Source: CAD feature listing. Evaluate the final solid. Frame: model axes, mm. Face numbers are marked on the shaded views. A direction names the side the tool comes from. Give positions to 0.01 mm unless a question says otherwise; leave off trailing zeros. Write each loop counter-clockwise with the first axis right and the second up, starting at its lowest first coordinate (ties: lowest second). Pieces come first, ordered by that corner, then holes. Notation, with made-up numbers: M 33.25,21 L 69.25,21 A31 cw 69.25,58 Z; hole C 23,32 d3. An arc over 180 degrees is marked long. Return JSON: item names as keys, results as strings.
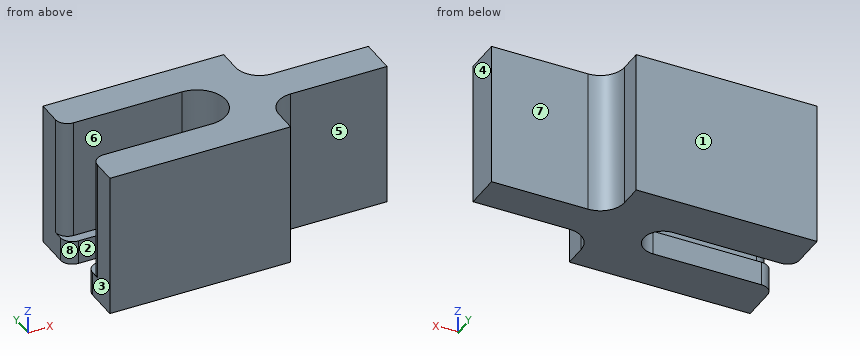
```python
from build123d import *

# Parameters (mm, degrees)
BOSS_EXTRUDE1_DEPTH      = 10
BOSS_EXTRUDE1_DEPTH_BACK = 2
BOSS_EXTRUDE2_START      = -2
BOSS_EXTRUDE2_DEPTH      = 2
FILLET6_R                = 1
FILLET7_R                = 1
BOSS_EXTRUDE3_DEPTH      = 10
BOSS_EXTRUDE3_DEPTH_BACK = 2
SKETCH1_5_W              = 7.906812167
SKETCH1_5_H              = 3
SKETCH1_5_W_2            = 2.093187833
FILLET8_R                = 2


with BuildPart() as part:
    # Sketch1 → Boss-Extrude1 (new, two sides: drawn at the far end of the back side and taken through both)
    with BuildSketch(Plane.XY.offset(-BOSS_EXTRUDE1_DEPTH_BACK)):
        with BuildLine():
            Line((-10, 2.4), (0, 2.4))
            ThreePointArc((0, 2.4), (2.4, 0), (0, -2.4))
            Line((0, -2.4), (-10, -2.4))
            Line((-10, -2.4), (-10, -5.4))
            Line((-10, -5.4), (5, -5.4))
            Line((5, -5.4), (5, -1.5))
            Line((5, -1.5), (5, 1.5))
            Line((5, 1.5), (5, 5.4))
            Line((5, 5.4), (-10, 5.4))
            Line((-10, 5.4), (-10, 2.4))
        make_face()
    extrude(amount=BOSS_EXTRUDE1_DEPTH + BOSS_EXTRUDE1_DEPTH_BACK)

    # Sketch1_4 → Boss-Extrude2 (add)
    with BuildSketch(Plane.XY.offset(BOSS_EXTRUDE2_START)):
        with BuildLine():
            Line((0, 1.6), (-10, 1.6))
            Line((-10, 1.6), (-10, 2.4))
            Line((-10, 2.4), (0, 2.4))
            ThreePointArc((0, 2.4), (2.4, 0), (0, -2.4))
            Line((0, -2.4), (-10, -2.4))
            Line((-10, -2.4), (-10, -1.6))
            Line((-10, -1.6), (0, -1.6))
            ThreePointArc((0, -1.6), (1.6, 0), (0, 1.6))
        make_face()
        with BuildLine():
            Line((-10, 2.4), (0, 2.4))
            ThreePointArc((0, 2.4), (2.4, 0), (0, -2.4))
            Line((0, -2.4), (-10, -2.4))
            Line((-10, -2.4), (-10, -5.4))
            Line((-10, -5.4), (5, -5.4))
            Line((5, -5.4), (5, -1.5))
            Line((5, -1.5), (5, 1.5))
            Line((5, 1.5), (5, 5.4))
            Line((5, 5.4), (-10, 5.4))
            Line((-10, 5.4), (-10, 2.4))
        make_face()
    extrude(amount=BOSS_EXTRUDE2_DEPTH)

    # Fillet6
    fillet6_edges = [part.edges().sort_by_distance(p)[0] for p in [
        (-10, -2.4, 5),
        (-10, 2.4, 5),
    ]]
    fillet(fillet6_edges, radius=FILLET6_R)

    # Fillet7
    fillet7_edges = [part.edges().sort_by_distance(p)[0] for p in [
        (-10, 1.6, -1),
        (-10, -1.6, -1),
    ]]
    fillet(fillet7_edges, radius=FILLET7_R)

    # Sketch1_5 → Boss-Extrude3 (add, two sides: drawn at the far end of the back side and taken through both)
    with BuildSketch(Plane.XY.offset(-BOSS_EXTRUDE3_DEPTH_BACK)):
        with Locations((8.953406083, 0)):
            Rectangle(SKETCH1_5_W, SKETCH1_5_H)
        with Locations((13.953406084, 0)):
            Rectangle(SKETCH1_5_W_2, SKETCH1_5_H)
    extrude(amount=BOSS_EXTRUDE3_DEPTH + BOSS_EXTRUDE3_DEPTH_BACK)

    # Fillet8
    fillet8_edges = [part.edges().sort_by_distance(p)[0] for p in [
        (5, -1.5, 4),
        (5, 1.5, 4),
    ]]
    fillet(fillet8_edges, radius=FILLET8_R)


solid = part.part
```
1) Cut plane D-D, the plane x = 13.75. Return the cut outline in (y, z), then the cut area to 3 significant figures.
Numbers:
{"outline": "M -1.5,-2 L 1.5,-2 L 1.5,10 L -1.5,10 Z", "area": "36.0 mm²"}
2) Cut plane A-A, the plane x = -0.5. Return the cut outline in (y, z), then the cut area to 3 significant figures.
Numbers:
{"outline": "M -5.4,-2 L -1.6,-2 L -1.6,0 L -2.4,0 L -2.4,10 L -5.4,10 Z; M 1.6,-2 L 5.4,-2 L 5.4,10 L 2.4,10 L 2.4,0 L 1.6,0 Z", "area": "75.2 mm²"}
3) Line query: line 1 (Y direction, x = -7.75, z = -1); line 2 (Y direction, x = -5, z = 8.75); line 3 (X direction, y = 4.75, z = 3). Output: solid intervals per line, ascending. Write a range as [from, to].
Numbers:
{"line 1": "y = [-5.4, -1.6], [1.6, 5.4]", "line 2": "y = [-5.4, -2.4], [2.4, 5.4]", "line 3": "x = [-10, 5]"}
4) Cut plane C-C, the plane z = 4. Return the cut outline in (x, y).
Numbers:
{"outline": "M -10,-5.4 L 5,-5.4 L 5,-3.5 A2 cw 7,-1.5 L 15,-1.5 L 15,1.5 L 7,1.5 A2 cw 5,3.5 L 5,5.4 L -10,5.4 L -10,3.4 A1 ccw -9,2.4 L 0,2.4 A2.4 cw 0,-2.4 L -9,-2.4 A1 ccw -10,-3.4 Z"}
5) Draft query along Y for the marked faces 1, 2 and 3. Return one class per face: released by +Y, released by -Y, zero draft, split by the parting line, or undercut.
Numbers:
{"face 1": "released by +Y", "face 2": "undercut", "face 3": "zero draft"}
6) Contact query for flat-ended pins moving along their axis: pin 1 Ø4 at (x, z) = (10, 4) entering from -Y; pin 2 Ø6.5 at (x, z) = (11.5, 4.5) entering from +Y; pin 3 Ø1.5 at (y, z) = (-4.5, 1) entering from +X. Output: stop coordinate, or through.
Numbers:
{"pin 1": "stops at y = -1.5", "pin 2": "stops at y = 1.5", "pin 3": "stops at x = 5"}
7) Cut plane B-B, the plane y = 0. Return the cut outline in (x, z), then the cut area to 3 significant figures.
Numbers:
{"outline": "M 1.6,-2 L 15,-2 L 15,10 L 2.4,10 L 2.4,0 L 1.6,0 Z", "area": "153 mm²"}
8) Set-up query: the marked faces 4, 5, 6, 7 and 8. Return all of +Z, -Z, +X, -X, +Y, -Y with unobstructed straight access to the full face (end or side cutting, diameter ignored); none if empty.
Numbers:
{"face 4": "+Z, -Z, +X, +Y, -Y", "face 5": "+Z, -Z, +X, -Y", "face 6": "+Z, -X", "face 7": "+Z, -Z, +X, +Y", "face 8": "+Z, -Z, -X"}
